Autodesk Fusion 360 part; units mm, degrees
sketch "Sketch1" plane through (0, 0, 0) normal (0, 1, 0) x (1, 0, 0)
  line L0 (6, 6) -> (-6, 6)
  line L1 (-6, 6) -> (-6, -6)
  line L2 (-6, -6) -> (6, -6)
  line L3 (6, -6) -> (6, 6)
  line L4 (6, 6) -> (-6, -6) construction
  line L5 (-6, 6) -> (6, -6) construction
  dimension "d1" = 12
  dimension "d2" = 12
extrude "Extrude1" add sketch "Sketch1" along normal blind 4 makes body 1
sketch "Sketch2" plane through (0, 4, 0) normal (0, 1, 0) x (-1, 0, 0)
  line L0 (-6, 6) -> (-6, -6)
  line L1 (-6, -6) -> (6, -6)
  line L2 (6, -6) -> (6, 6)
  line L3 (6, 6) -> (-6, 6)
  circle A0 centre (0, 0) radius 3.375
  line L4 (-3, -3.5) -> (3, -3.5)
  line L5 (3, -3.5) -> (3, 3.5)
  line L6 (3, 3.5) -> (-3, 3.5)
  line L7 (-3, 3.5) -> (-3, -3.5)
  line L8 (-3, -3.5) -> (3, 3.5) construction
  line L9 (3, -3.5) -> (-3, 3.5) construction
  dimension "d5" = 6.75
  dimension "d6" = 6
  dimension "d7" = 7
extrude "Extrude2" cut sketch "Sketch2" against normal blind 5 contours A0 L5 L7 bodies 1
sketch "Sketch3" plane through (0, 0, 0) normal (0, -1, 0) x (1, 0, 0)
  line L0 (3, 1.5462) -> (3, -1.5462)
  arc A0 (-3, -1.5462) -> (3, -1.5462) centre (0, 0) ccw
  line L1 (-3, -1.5462) -> (-3, 1.5462)
  arc A1 (3, 1.5462) -> (-3, 1.5462) centre (0, 0) ccw
  line L2 (6, -6) -> (6, 6)
  line L3 (6, 6) -> (-6, 6)
  line L4 (-6, 6) -> (-6, -6)
  line L5 (-6, -6) -> (6, -6)
  line L6 (6, 7.5) -> (-6, 7.5)
  line L7 (-6, 7.5) -> (-6, -7.5)
  line L8 (-6, -7.5) -> (6, -7.5)
  line L9 (6, -7.5) -> (6, 7.5)
  line L10 (6, 7.5) -> (-6, -7.5) construction
  line L11 (-6, 7.5) -> (6, -7.5) construction
  dimension "d10" = 12
  dimension "d11" = 15
extrude "Extrude3" add sketch "Sketch3" against normal blind 4 separate body contours L5 L7 L8 L9 | L3 L6 L7 L9 makes body 2 at (2, 1.3333, 6) makes body 3 at (-2, 1.3333, -7.5)
sketch "Sketch4" plane through (0, 0, 0) normal (0, -1, 0) x (1, 0, 0)
  line L0 (3, 1.5462) -> (3, -1.5462)
  arc A0 (-3, -1.5462) -> (3, -1.5462) centre (0, 0) ccw
  line L1 (-3, -1.5462) -> (-3, 1.5462)
  arc A1 (3, 1.5462) -> (-3, 1.5462) centre (0, 0) ccw
  line L2 (6, -6) -> (6, 6)
  line L3 (6, 6) -> (-6, 6)
  line L4 (-6, 6) -> (-6, -6)
  line L5 (-6, -6) -> (6, -6)
  line L6 (6, 6) -> (-6, 6)
  line L7 (-6, 6) -> (-6, -6)
  line L8 (-6, -6) -> (6, -6)
  line L9 (6, -6) -> (6, 6)
  line L10 (6, 6) -> (-6, -6) construction
  line L11 (-6, 6) -> (6, -6) construction
  dimension "d14" = 12
  dimension "d15" = 12
extrude "Extrude4" add sketch "Sketch4" along normal blind 5 bodies 1 2 3
sketch "Sketch5" plane through (0, -5, 0) normal (0, -1, 0) x (1, 0, 0)
  arc A0 (-3, -1.5462) -> (3, -1.5462) centre (0, 0) ccw
  line L0 (-3, -1.5462) -> (-3, 1.5462)
  arc A1 (3, 1.5462) -> (-3, 1.5462) centre (0, 0) ccw
  line L1 (3, 1.5462) -> (3, -1.5462)
  line L2 (6, -6) -> (6, 6)
  line L3 (6, 6) -> (-6, 6)
  line L4 (-6, 6) -> (-6, -6)
  line L5 (-6, -6) -> (6, -6)
  line L6 (5, 5.6) -> (-5, 5.6)
  line L7 (-5, 5.6) -> (-5, -5.6)
  line L8 (-5, -5.6) -> (5, -5.6)
  line L9 (5, -5.6) -> (5, 5.6)
  line L10 (5, 5.6) -> (-5, -5.6) construction
  line L11 (-5, 5.6) -> (5, -5.6) construction
  dimension "d18" = 11.2
Geometry check sheet. Reference: the model listing, model coordinates, mm. A direction names the side the tool comes from. Coordinates: 2 decimals unless noted, no trailing zeros. Order: outer loops, then holes, each group sorted by start corner. A loop starts at its lowest first (then second) coordinate and runs counter-clockwise, first axis right, second up. Notation, with made-up numbers: M 44,51.5 L 73,51.5 A35 ccw 73,87.5 Z; hole C -16,56 d6. An arc over 180 degrees is marked long. One line per question, with ' | ' between items. Start each with the question number.
Item 1: Cross-section at C-C on y = 1.75. Enter the section's corners in (x, z) (3 decimals), then the cut area to 3 significant figures.
Item 2: Cross-section at B-B on z = 1.25. Enter the section's corners in (x, y).
Item 3: Cross-section at D-D on x = 5. Enter the section's corners in (y, z), then the cut area to 3 significant figures.
Item 4: Set-up check for faces 5 (the flat face through (0, 2, 7.5)), 6 (the flat face through (3, -5, 3)), 7 (the flat face through (0, 0, -7)), 8 (the flat face through (0, -2, 6)), 9 (the cylindrical face through (-0.052, 2.028, 3.375)): record each of +Z, -Z, +X, -X, +Y, -Y from which the full face is reachable in a straight line by a thin tool's end or side.
Item 5: Material ranges on L1, parallel to Z at x = 0, y = 2 (3 decimals); L2, parallel to X at y = 0.25, z = 3; L3, parallel to Z at x = -4, y = -3.75, recorded low to high. Write a range as [from, to].
Item 6: Gauge pin test, flat ends, axial feed: pin 1 (2 mm diameter, centred on x = 0, y = -3, fed in from -Z); pin 2 (1.5 mm diameter, centred on x = 0.5, z = 0, fed in from -Y); pin 3 (4 mm diameter, centred on x = -0.5, y = -2.5, fed in from +Z). Record the tip position at first contact, or that the pin passes through.
Item 7: Cross-section at A-A on x = 0. Enter the section's corners in (y, z) (3 decimals), then the cut area to 4 significant figures.
Item 8: Draft check along X on faces 1 (the flat face through (3, 0, 0)), 2 (the cylindrical face through (-0.052, -2.465, 3.375)), 3 (the flat face through (-6, -1, 0)), 4 (the flat face through (0, 0, 7)). Enter one of: pulls with the +X half, pulls with the -X half, needs draft (parallel to the pull), parting line crosses it, or undercut.
Findings:
1) outline: M -6,-7.5 L 6,-7.5 L 6,7.5 L -6,7.5 Z; hole M -3,-1.546 A3.375 ccw 3,-1.546 L 3,1.546 A3.375 ccw -3,1.546 Z | area: 146 mm²
2) outline: M -6,-5 L -3,-5 L -3,4 L -6,4 Z; M 3,-5 L 6,-5 L 6,4 L 3,4 Z
3) outline: M -5,-6 L 0,-6 L 0,-7.5 L 4,-7.5 L 4,7.5 L 0,7.5 L 0,6 L -5,6 Z | area: 120 mm²
4) face 5: +Z, +X, -X, +Y, -Y | face 6: +Z, -Z, +X, -X, -Y | face 7: -Z, +X, -X, -Y | face 8: +Z, +X, -X, -Y | face 9: +Y, -Y
5) L1: z = [-7.5, -3.375], [3.375, 7.5] | L2: x = [-6, -1.55], [1.55, 6] | L3: z = [-6, 6]
6) pin 1: stops at z = -6 | pin 2: passes through | pin 3: stops at z = 6
7) outline: M -5,-6 L 0,-6 L 0,-7.5 L 4,-7.5 L 4,-3.375 L -5,-3.375 Z; M -5,3.375 L 4,3.375 L 4,7.5 L 0,7.5 L 0,6 L -5,6 Z | area: 59.25 mm²
8) face 1: undercut | face 2: undercut | face 3: pulls with the -X half | face 4: needs draft
